The figure shows three views and two pictorial views of one solid part (mm, origin at its lowest corner). Answer the questions. A direction names the side the tool comes from. Coordinates: 2 decimals unless noted, no trailing zeros. Write each loop counter-clockwise with the first axis right and the second up, starting at its lowest first coordinate (ties: lowest second). Pieces come first, ordered by that corner, then holes.
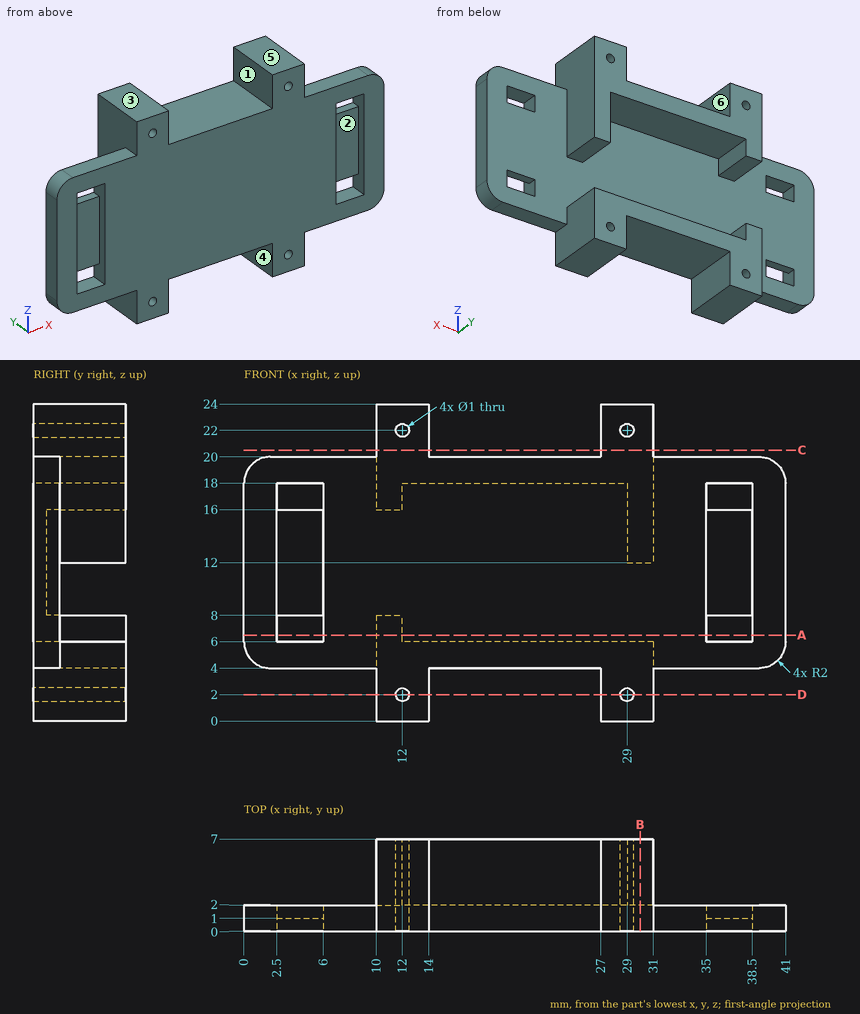
Q1. The part is cut by section D-D, the plane z = 2. Write down the section's boundary in (x, y).
Answers below:
outline: (10, 0) - (11.5, 0) - (11.5, 7) - (10, 7) - close; (12.5, 0) - (14, 0) - (14, 7) - (12.5, 7) - close; (27, 0) - (28.5, 0) - (28.5, 7) - (27, 7) - close; (29.5, 0) - (31, 0) - (31, 7) - (29.5, 7) - close
Q2. The part is cut by section B-B, the plane x = 30. Write down the section's boundary in (y, z).
Answers below:
outline: (0, 0) - (7, 0) - (7, 6) - (2, 6) - (2, 12) - (7, 12) - (7, 24) - (0, 24) - close
Q3. Given pin 1 (10 mm diameter, centred on x = 11, z = 16, fed in from -Y); pin 2 (4 mm diameter, centred on y = 4.5, z = 2.5, fed in from +X); pin 3 (2 mm diameter, centred on x = 22.5, y = 2, fed in from -Z); pin 4 (1.1 mm diameter, centred on x = 36.5, y = 1.5, fed in from +Z), each flat-ended and moving along its own axis, determine where each tip first touches the part or whether it passes through.
Answers below:
pin 1: stops at y = 0
pin 2: stops at x = 31
pin 3: stops at z = 4
pin 4: stops at z = 20
Q4. Find the intervals of material crossed by probe 1 along X at (y, z) = (2.5, 2); probe 2 along X at (y, z) = (2, 23.25); probe 3 along Z at (x, y) = (17, 6.25), in increasing order.
Answers below:
probe 1: x = 10 to 11.5, 12.5 to 14, 27 to 28.5, 29.5 to 31
probe 2: x = 10 to 14, 27 to 31
probe 3: z = 4 to 6, 18 to 20
Q5. Which of the six approach directions +Z, -Z, +X, -X, +Y, -Y give full straight-line access (tool end or side, diameter ignored) to the marked faces 1, 2, 3 and 4?
Answers below:
face 1: +Z, +Y, -Y
face 2: -Y
face 3: +Z, +X, -X, +Y, -Y
face 4: -Z, +Y, -Y
Q6. The part is cut by section A-A, the plane z = 6.5. Write down the section's boundary in (x, y).
Answers below:
outline: (0, 0) - (2.5, 0) - (2.5, 2) - (0, 2) - close; (6, 0) - (35, 0) - (35, 2) - (12, 2) - (12, 7) - (10, 7) - (10, 2) - (6, 2) - close; (38.5, 0) - (41, 0) - (41, 2) - (38.5, 2) - close
Q7. Determine the mould class of the marked faces 5 and 6 for opening direction X: released by +X, released by -X, zero draft, split by the parting line, or undercut.
Answers below:
face 5: zero draft
face 6: undercut
Q8. The part is cut by section C-C, the plane z = 20.5. Write down the section's boundary in (x, y).
Answers below:
outline: (10, 0) - (14, 0) - (14, 7) - (10, 7) - close; (27, 0) - (31, 0) - (31, 7) - (27, 7) - close
